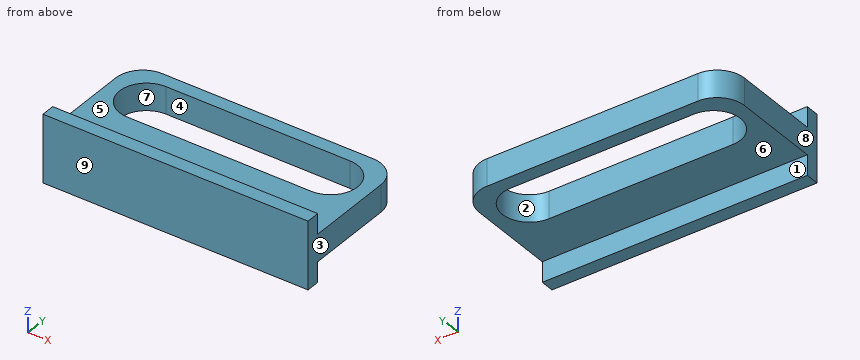
Autodesk Inventor part; units mm, degrees
ref_plane "YZ Plane" through (0, 0, 0) normal (1, 0, 0) x (0, 1, 0)
ref_plane "XZ Plane" through (0, 0, 0) normal (0, 1, 0) x (-1, 0, 0)
ref_plane "XY Plane" through (0, 0, 0) normal (0, 0, 1) x (1, 0, 0)
sketch "Sketch1" plane through (0, 0, 0) normal (0, 0, 1) x (1, 0, 0)
  line L0 (0, 0) -> (68.1, 0)
  circle A0 centre (0, 0) radius 10
  circle A1 centre (68.1, 0) radius 10
  line L1 (0, 10) -> (68.1, 10)
  line L2 (0, -10) -> (68.1, -10)
  circle A2 centre (0, 0) radius 15
  circle A3 centre (68.1, 0) radius 15
  line L3 (0, 15) -> (68.1, 15)
  line L4 (68.1, -15) -> (0, -15)
  dimension "d0" = 68.1
  dimension "d1" = 20
  dimension "d2" = 20
  dimension "d3" = 30
  dimension "d4" = 30
extrude "Extrusion1" add sketch "Sketch1" along normal blind 10 contours A0 L2 A2 L1 | A2 L3 A3 L1 | L2 A3 L4 A2 | A3 L2 A1 L1
sketch "Sketch2" plane through (0, 0, 10) normal (0, 0, 1) x (1, 0, 0)
  line L0 (0, 0) -> (0, -32.5) construction
  arc A0 (0, 15) -> (0, -15) centre (0, 0) ccw construction
  line L1 (-15, 0) -> (-15, -32.5) construction
  arc A1 (68.1, -15) -> (68.1, 15) centre (68.1, 0) ccw construction
  line L2 (83.1, 0) -> (83.1, -32.5) construction
  line L3 (-15, -32.5) -> (-15, 15)
  line L4 (-15, 15) -> (83.1, 15)
  line L5 (83.1, 15) -> (83.1, -32.5)
  line L6 (83.1, -32.5) -> (-15, -32.5)
  line L7 (0, 10) -> (68.1, 10)
  arc A2 (0, 10) -> (0, -10) centre (0, 0) ccw
  line L8 (68.1, -10) -> (0, -10)
  arc A3 (68.1, -10) -> (68.1, 10) centre (68.1, 0) ccw
  dimension "d7" = 32.5
extrude "Extrusion2" add sketch "Sketch2" against normal blind 10
fillet "Fillet1" radius 10 1 edges at (83.1, 15, 5)
fillet "Fillet2" radius 10 1 edges at (-15, 15, 5)
ref_plane "Work Plane1" through (0, 0, 5) normal (0, 0, 1) x (1, 0, 0)
sketch "Sketch3" plane through (0, 0, 5) normal (0, 0, 1) x (1, 0, 0)
  arc A0 (-5, 15) -> (-15, 5) centre (-5, 5) ccw
  line L0 (-5, 15) -> (73.1, 15)
  line L1 (83.1, 5) -> (83.1, -32.5)
  line L2 (83.1, -32.5) -> (-15, -32.5)
  line L3 (-15, -32.5) -> (-15, 5)
  line L4 (0, 10) -> (68.1, 10)
  arc A1 (0, 10) -> (0, -10) centre (0, 0) ccw
  line L5 (68.1, -10) -> (0, -10)
  arc A2 (68.1, -10) -> (68.1, 10) centre (68.1, 0) ccw
  line L6 (83.1, -32.5) -> (-15, -32.5)
  line L7 (-15, -32.5) -> (83.1, -32.5)
  line L8 (83.1, -32.5) -> (83.1, -27.5)
  line L9 (83.1, -27.5) -> (-15, -27.5)
  line L10 (-15, -27.5) -> (-15, -32.5)
  arc A3 (83.1, 5) -> (73.1, 15) centre (73.1, 5) ccw
  dimension "d12" = 5
extrude "Extrusion3" add sketch "Sketch3" along normal mid plane 25 contours L9 L1 L2 L3
ref_plane "Work Plane2" through (68.1, -10, 10) normal (1, 0, 0) x (0, 0, -1)
ref_plane "Work Plane3" through (0, -10, 10) normal (1, 0, 0) x (0, 0, -1)
ref_plane "Work Plane4" through (34.05, 5, 10) normal (1, 0, 0) x (0, 0, -1)
properties part number "PistaEslabonPreliminar"
Design review of the part built by this model. Coordinates are the model's own, in mm. Face numbers are marked on the shaded views. A direction names the side the tool comes from. Round coordinates to 2 decimals unless told otherwise and drop trailing zeros. Order: outer loops, then holes, each group sorted by start corner. A loop starts at its lowest first (then second) coordinate and runs counter-clockwise, first axis right, second up.
1) For L1, parallel to Y at x = 21, z = 7.25; L2, parallel to Y at x = 20.5, z = -5; L3, parallel to Z at x = 3, y = -17.5, list the stretches that pass through material, from the lowest coordinate up.
The answers:
L1: y = -32.5 to -10, 10 to 15
L2: y = -32.5 to -27.5
L3: z = 0 to 10
2) Consider section B-B (x = 44). State the section outline as (y, z) points, plus the area to 3 significant figures.
The answers:
outline: (-32.5, -7.5) - (-27.5, -7.5) - (-27.5, 0) - (-10, 0) - (-10, 10) - (-27.5, 10) - (-27.5, 17.5) - (-32.5, 17.5) - close; (10, 0) - (15, 0) - (15, 10) - (10, 10) - close
area: 350 mm2
3) Consider section A-A (y = 0). State the section outline as (x, z) points, plus the area to 3 significant figures.
The answers:
outline: (-15, 0) - (-10, 0) - (-10, 10) - (-15, 10) - close; (78.1, 0) - (83.1, 0) - (83.1, 10) - (78.1, 10) - close
area: 100 mm2
4) Consider section C-C (z = 6.75). State the section outline as (x, y) points, plus the area to 3 significant figures.
The answers:
outline: (-15, -32.5) - (83.1, -32.5) - (83.1, 5) arc R10 ccw to (73.1, 15) - (-5, 15) arc R10 ccw to (-15, 5) - close; hole (0, -10) - (68.1, -10) arc R10 ccw to (68.1, 10) - (0, 10) arc R10 ccw to start
area: 2,940 mm2
5) Machinability: for the marked faces 5, 6, 7, 8 and 9, which of the approach directions +Z, -Z, +X, -X, +Y, -Y give a long, thin tool a straight path to every point of the face, cutting with its end or side? Answer none if there is none.
The answers:
face 5: +Z, +X, -X, +Y
face 6: -Z, +X, -X, +Y
face 7: +Z, -Z
face 8: +Z, -Z, -X, +Y, -Y
face 9: +Z, -Z, +X, -X, -Y
6) Draft analysis for pull direction Y (two halves, no side actions). For the marked faces 1, 2, 3 and 4, state which applies: released by +Y, released by -Y, zero draft, split by the parting line, or undercut.
The answers:
face 1: released by +Y
face 2: undercut
face 3: zero draft
face 4: undercut
7) Clearance check with flat-ended pins moving along their axes: pin 1 Ø2 at (x, z) = (16, 14) entering from +Y; pin 2 Ø10 at (x, y) = (34, 1) entering from -Z (3 decimals); pin 3 Ø5 at (y, z) = (8.5, 2.5) entering from -X; pin 4 Ø2 at (x, y) = (33.5, -23) entering from +Z. State where each tip first meets the part, or that it passes through.
The answers:
pin 1: stops at y = -27.5
pin 2: passes through
pin 3: stops at x = -14.95
pin 4: stops at z = 10
8) Consider section D-D (z = -5). State the section outline as (x, y) points.
The answers:
outline: (-15, -32.5) - (83.1, -32.5) - (83.1, -27.5) - (-15, -27.5) - close
